Can you work these out from the model? Positions are in its coordinate system, mm. A direction names the side the tool comes from. Round coordinates to 2 decimals unless told otherwise and drop trailing zeros. Order: outer loops, then holes, each group sorted by start corner. A loop starts at its lowest first (then second) coordinate and runs counter-clockwise, first axis right, second up.
Q1. We'd pull the mould along Z, two halves only. Please class faces 3 (the face through (49, -6, 1.439)), 4 (the face through (49, 0, 27)), 5 (the face through (171.12, -6.44, 19.06)), 6 (the face through (52, -6, 52.239)): pulls with the +Z half, pulls with the -Z half, needs draft (parallel to the pull), parting line crosses it, or undercut.
Q2. Will these pins go through, and if not, where does the flat tip stop? P1, Ø12, axis at y = -5.5, z = 12.5, coming from the +X side; P2, Ø5, axis at y = -19, z = 46.5, coming from the -X side; P3, Ø8, axis at y = -19, z = 46, coming from the +X side.
Q3. If we section it at A-A (z = 11): Please give me the cut outline in (x, y).
Q4. If we section it at D-D (z = 44): Please give me the cut outline in (x, y), plus the area to 3 significant figures.
Q5. If we section it at B-B (y = -9): Please give me the cut outline in (x, z), plus the area to 3 significant figures.
Q6. If I drill on line 1 (Y direction, x = 24, z = 39); line 2 (X direction, y = -7, z = 14.5); line 3 (X direction, y = -3.5, z = 48.5), over which ranges is the centre line in solid material (lowest first)?
Q7. If we section it at C-C (x = -57): Please give me the cut outline in (y, z), plus the area to 3 significant figures.
Q8. For faces 1 (the face through (-51, -25.4, 27)), 2 (the face through (-53.496, -18.961, 46.986)), which set-ups out of +Z, -Z, +X, -X, +Y, -Y let a thin tool reach every point of the face, with its end or its side?
from build123d import *

# Parameters (mm, degrees)
F2_DEPTH = 12.7
F3_R     = 20.32
F4_DEPTH = 12.7
F5_DEPTH = 12.7


# Not quite as in the source:
# - a variable given as a bare number and used for a length is read in inches; the dataset says mm whatever the document's units were


with BuildPart() as f2:
    # F1 (on Front) → F2 (new body)
    with BuildSketch(Plane.XZ):
        with BuildLine():
            Line((152.3496784632, 52.2385248174), (-50.8503215368, 52.2385248174))
            ThreePointArc((-50.8503215368, 52.2385248174), (-68.8108337789, 44.7990370595), (-76.2503215368, 26.8385248174))
            ThreePointArc((-76.2503215368, 26.8385248174), (-68.8108337789, 8.8780125752), (-50.8503215368, 1.4385248174))
            Line((-50.8503215368, 1.4385248174), (152.3496784632, 1.4385248174))
            ThreePointArc((152.3496784632, 1.4385248174), (170.3101907054, 8.8780125752), (177.7496784632, 26.8385248174))
            ThreePointArc((177.7496784632, 26.8385248174), (170.3101907054, 44.7990370595), (152.3496784632, 52.2385248174))
        make_face()
    extrude(amount=F2_DEPTH)

    # F3 (on face) → F4 (join)
    with BuildSketch(Plane.XZ.offset(12.7)):
        with Locations((-50.8503215368, 26.8385248174)):
            Circle(F3_R)
    extrude(amount=F4_DEPTH)

    # F3 (on face) → F5 (cut)
    with BuildSketch(Plane.XZ.offset(12.7)):
        with Locations((152.3496784632, 26.8385248174)):
            Circle(F3_R)
    extrude(amount=-F5_DEPTH, mode=Mode.SUBTRACT)


solid = f2.part
Solution:
1. face 3: pulls with the -Z half
1. face 4: needs draft
1. face 5: undercut
1. face 6: pulls with the +Z half
2. P1: stops at x = 176.34
2. P2: stops at x = -61.73
2. P3: stops at x = -37.32
3. outline: (-70.71, -12.7) - (-63.58, -12.7) - (-63.58, -25.4) - (-38.12, -25.4) - (-38.12, -12.7) - (139.62, -12.7) - (139.62, 0) - (-70.71, 0) - close; (165.08, -12.7) - (172.21, -12.7) - (172.21, 0) - (165.08, 0) - close
4. outline: (-69.58, -12.7) - (-61.73, -12.7) - (-61.73, -25.4) - (-39.97, -25.4) - (-39.97, -12.7) - (141.47, -12.7) - (141.47, 0) - (-69.58, 0) - close; (163.23, -12.7) - (171.08, -12.7) - (171.08, 0) - (163.23, 0) - close
4. area: 3,060 mm2
5. outline: (-50.85, 1.44) - (152.35, 1.44) arc R25.4 ccw to (152.35, 52.24) - (-50.85, 52.24) arc R25.4 ccw to start; hole circle Ø40.64 at (152.35, 26.84)
5. area: 11,100 mm2
6. line 1: y = -12.7 to 0
6. line 2: x = -73.05 to 136.2, 168.49 to 174.55
6. line 3: x = -64.11 to 165.61
7. outline: (-25.4, 7.47) - (-12.7, 7.47) - (-12.7, 2.19) - (0, 2.19) - (0, 51.48) - (-12.7, 51.48) - (-12.7, 46.21) - (-25.4, 46.21) - close
7. area: 1,120 mm2
8. face 1: +Z, -Z, +X, -X, -Y
8. face 2: -Y
